Part print with two shaded views. Sizes in mm from the minimum x, y, z corner. Give positions to 0.01 mm unless a question says otherwise; leave off trailing zeros. Write each loop counter-clockwise with the first axis right and the second up, starting at its lowest first coordinate (ties: lowest second). Pieces come first, ordered by that corner, then holes.
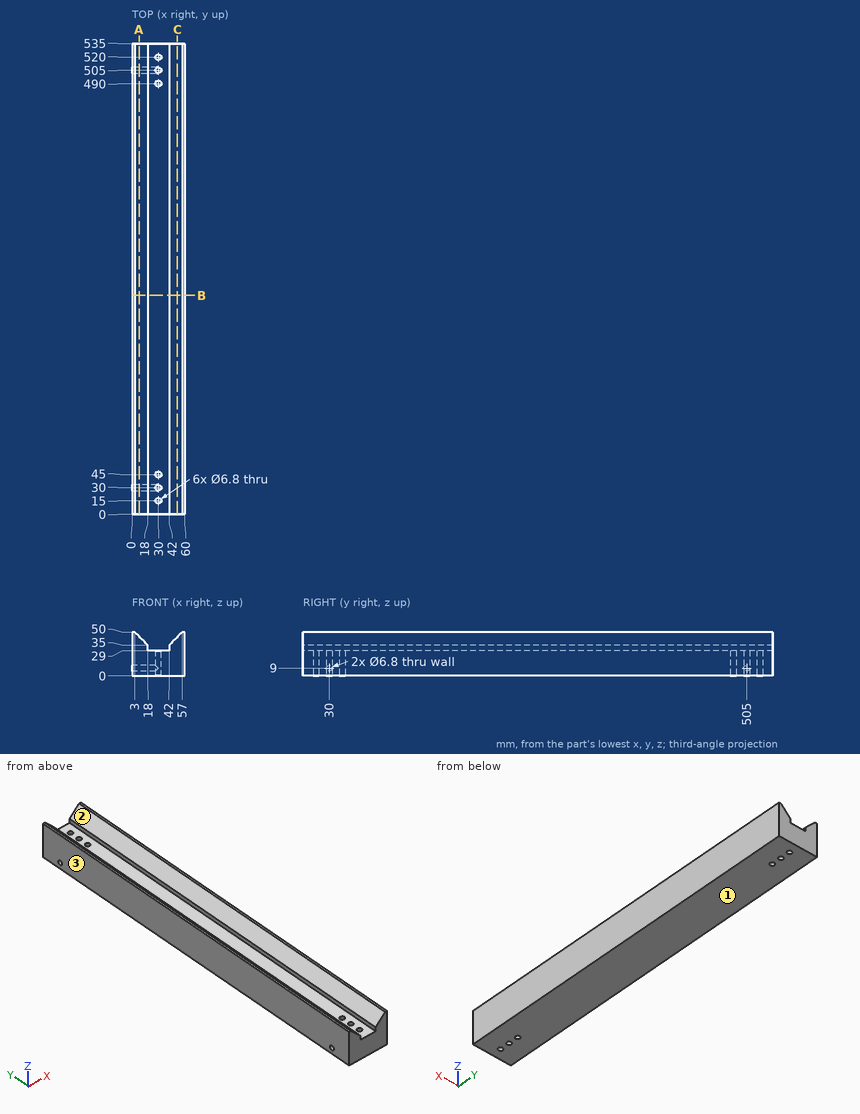
(1) Saw through at C-C, the plane x = 51.5. List the corners of the cut face in (y, z), plus the area to 3 significant figures.
(2) Saw through at B-B, the plane y = 249. List the corners of the cut face in (x, z).
(3) Saw through at A-A, the plane x = 8. List the corners of the cut face in (y, z), plus the area to 3 significant figures.
(4) Drop flat-ended pins along their axis: pin 1 (10 mm diameter, centred on x = 9.5, y = 392.5, fed in from +Z); pin 2 (2 mm diameter, centred on x = 10.5, y = 79, fed in from +Z); pin 3 (5.5 mm diameter, centred on x = 30, y = 505, fed in from +Z); pin 4 (9 mm diameter, centred on x = 30, y = 520, fed in from +Z). Give the stop position or say it passes through.
(5) Mould opens along X. For the marked faces 1, 2 and 3 say: +X half, -X half, draft (parallel to the pull), parting line (faces both ways), or undercut.
(6) Probe line 1 (X direction, y = 30, z = 19); line 2 (Z direction, x = 22, y = 30); line 3 (X direction, y = 137, z = 43.5). List the from-to ranges inside material, lowest first.
Computed values:
1. outline: (0, 0) - (535, 0) - (535, 44.5) - (0, 44.5) - close
1. area: 23,800 mm2
2. outline: (0, 0) - (60, 0) - (60, 50) - (57, 50) - (42, 35) - (42, 29) - (18, 29) - (18, 35) - (3, 50) - (0, 50) - close
3. outline: (0, 0) - (535, 0) - (535, 45) - (0, 45) - close; hole circle Ø6.8 at (30, 9); hole circle Ø6.8 at (505, 9)
3. area: 24,000 mm2
4. pin 1: stops at z = 48.5
4. pin 2: stops at z = 43.5
4. pin 3: passes through
4. pin 4: stops at z = 29
5. face 1: draft
5. face 2: undercut
5. face 3: -X half
6. line 1: x = 0 to 26.6, 33.4 to 60
6. line 2: z = 0 to 5.6, 12.4 to 29
6. line 3: x = 0 to 9.5, 50.5 to 60
